The model under review builds one solid part; all positions refer to its coordinate system, in mm. A direction names the side the tool comes from. Round coordinates to 2 decimals unless told otherwise and drop trailing zeros. Loops run counter-clockwise (first coordinate to the right, second up) from the corner with the lowest first, then second, coordinate; pieces in that order, holes last. Notation, with made-up numbers: M 22.5,60.25 L 63.5,60.25 A21 ccw 63.5,65.25 Z; hole C 39.5,63 d6. An arc over 180 degrees is marked long. One line per question, with ' | ' between items.
from build123d import *

# Parameters (mm, degrees)
CROQUIS1_R              = 3.5
CROQUIS1_R_2            = 2.65
CROQUIS1_R_3            = 3.7
SALIENTE_EXTRUIR2_DEPTH = 8


with BuildPart() as part:
    # Croquis1 → Saliente-Extruir2 (new body)
    with BuildSketch(Plane(origin=(0, 0, 0), x_dir=(1, 0, 0), z_dir=(0, 1, 0))):
        with BuildLine():
            ThreePointArc((40, -30), (38.535533906, -33.535533906), (35, -35))
            Line((35, -35), (-35, -35))
            ThreePointArc((-35, -35), (-38.535533906, -33.535533906), (-40, -30))
            Line((-40, -30), (-40, 30))
            ThreePointArc((-40, 30), (-38.535533906, 33.535533906), (-35, 35))
            Line((-35, 35), (35, 35))
            ThreePointArc((35, 35), (38.535533906, 33.535533906), (40, 30))
            Line((40, 30), (40, -30))
        make_face()
        with Locations((31.259169622, 0)):
            Circle(CROQUIS1_R, mode=Mode.SUBTRACT)
        with Locations((30.25001, 25)):
            Circle(CROQUIS1_R_2, mode=Mode.SUBTRACT)
        with Locations((30.25001, -25)):
            Circle(CROQUIS1_R_2, mode=Mode.SUBTRACT)
        with Locations((-31.263846279, 0)):
            Circle(CROQUIS1_R, mode=Mode.SUBTRACT)
        with Locations((-30.264120004, 24.99741)):
            Circle(CROQUIS1_R_3, mode=Mode.SUBTRACT)
        with Locations((-30.264120004, -25.00224)):
            Circle(CROQUIS1_R_3, mode=Mode.SUBTRACT)
        with BuildLine():
            ThreePointArc((19.5, -17.5), (21.621320344, -16.621320344), (22.5, -14.5))
            Line((22.5, -14.5), (22.5, 14.5))
            ThreePointArc((22.5, 14.5), (21.621320344, 16.621320344), (19.5, 17.5))
            Line((19.5, 17.5), (-19.5, 17.5))
            ThreePointArc((-19.5, 17.5), (-21.621320344, 16.621320344), (-22.5, 14.5))
            Line((-22.5, 14.5), (-22.5, -14.5))
            ThreePointArc((-22.5, -14.5), (-21.621320344, -16.621320344), (-19.5, -17.5))
            Line((-19.5, -17.5), (19.5, -17.5))
        make_face(mode=Mode.SUBTRACT)
    extrude(amount=SALIENTE_EXTRUIR2_DEPTH)


solid = part.part
1) Add section C-C on z = 0. State the section outline as (x, y) points.
Output values:
outline: M -40,0 L -34.76,0 L -34.76,8 L -40,8 Z; M -27.76,0 L -22.5,0 L -22.5,8 L -27.76,8 Z; M 22.5,0 L 27.76,0 L 27.76,8 L 22.5,8 Z; M 34.76,0 L 40,0 L 40,8 L 34.76,8 Z
2) Add section D-D on y = 1.75. State the section outline as (x, z) points.
Output values:
outline: M -40,-30 A5 ccw -35,-35 L 35,-35 A5 ccw 40,-30 L 40,30 A5 ccw 35,35 L -35,35 A5 ccw -40,30 Z; hole C -31.26,0 d7; hole C -30.26,-25 d7.4; hole C -30.26,25 d7.4; hole M -22.5,-14.5 A3 ccw -19.5,-17.5 L 19.5,-17.5 A3 ccw 22.5,-14.5 L 22.5,14.5 A3 ccw 19.5,17.5 L -19.5,17.5 A3 ccw -22.5,14.5 Z; hole C 30.25,-25 d5.3; hole C 30.25,25 d5.3; hole C 31.26,0 d7
3) Add section B-B on z = -11. State the section outline as (x, y) points.
Output values:
outline: M -40,0 L -22.5,0 L -22.5,8 L -40,8 Z; M 22.5,0 L 40,0 L 40,8 L 22.5,8 Z
4) For line 1 (X direction, y = 4.25, z = 0); line 2 (X direction, y = 3.5, z = 25); line 3 (X direction, y = 0.5, z = -15.5), list the stretches that pass through material, from the lowest coordinate up.
Output values:
line 1: x = -40 to -34.76, -27.76 to -22.5, 22.5 to 27.76, 34.76 to 40 | line 2: x = -40 to -33.96, -26.56 to 27.6, 32.9 to 40 | line 3: x = -40 to -22.33, 22.33 to 40
5) Add section A-A on x = -8.5. State the section outline as (y, z) points.
Output values:
outline: M 0,-35 L 8,-35 L 8,-17.5 L 0,-17.5 Z; M 0,17.5 L 8,17.5 L 8,35 L 0,35 Z
6) Mouldability with a two-part tool opening along X and no side actions: class faces 1 (the cylindrical face through (39, 4, 33)), 2 (the cylindrical face through (27.763, 3.944, -0.154)), 3 (the flat face through (0, 4, -35)) as +X half, -X half, draft (parallel to the pull), parting line (faces both ways), or undercut.
Output values:
face 1: +X half | face 2: undercut | face 3: draft
7) Machinability: for faces 4 (the flat face through (0, 4, 35)), 5 (the cylindrical face through (-21.64, 3.94, 16.6)), which of the approach directions +Z, -Z, +X, -X, +Y, -Y give a long, thin tool a straight path to every point of the face, cutting with its end or side? Answer none if there is none.
Output values:
face 4: +Z, +X, -X, +Y, -Y | face 5: +Y, -Y
8) Insertion check: P1, Ø6, axis at x = -30.26, z = 25, coming from the -Y side. The pin has a flat end and moves straight along its axis. Give the tip position at first contact, or say it passes through.
Output values:
P1: passes through
